Source: CAD feature listing. Evaluate the final solid. Frame: model axes, mm. Give positions to 0.01 mm unless a question says otherwise; leave off trailing zeros. Loops run counter-clockwise (first coordinate to the right, second up) from the corner with the lowest first, then second, coordinate; pieces in that order, holes last. Notation, with made-up numbers: M 45,-13.75 L 56,-13.75 A12 ccw 56,1.25 Z; hole C 50,-2 d11. An arc over 180 degrees is marked long. Put each result on its own line as item: value. Start each with the question number.
```python
from build123d import *

# Parameters (mm, degrees)
SKETCH1_R           = 3.5
BOSS_EXTRUDE1_DEPTH = 15
BOSS_EXTRUDE1_TAPER = 4


with BuildPart() as part:
    # Sketch1 → Boss-Extrude1 (new body)
    with BuildSketch(Plane(origin=(0, 0, 0), x_dir=(0, 0, -1), z_dir=(1, 0, 0))):
        Circle(SKETCH1_R)
    extrude(amount=BOSS_EXTRUDE1_DEPTH, taper=BOSS_EXTRUDE1_TAPER)

    # Sketch2 → Revolve1 (revolve)
    with BuildSketch(Plane(origin=(16, 0, 0), x_dir=(0, 0, -1), z_dir=(1, 0, 0))):
        with BuildLine():
            Line((0, 2.451097821), (0, -2.451097821))
            ThreePointArc((0, -2.451097821), (2.451097821, 0), (0, 2.451097821))
        make_face()
    revolve(axis=Axis((16, 2.451097821, 0), (0, -1, 0)))


solid = part.part
```
1. Section B-B, the plane x = 10.75. Output: boundary loops of the cut face in (y, z), plus the area to 3 significant figures.
2. Section A-A, the plane z = 0. Output: boundary loops of the cut face in (x, y).
3. Ray query, line 1 (Z direction, x = 4.75, y = 2); line 2 (Z direction, x = 2.5, y = -0.25); line 3 (Y direction, x = 15.75, z = 2). Return the intervals inside material, ascending.
4. Section C-C, the plane x = 4.25. Output: boundary loops of the cut face in (y, z), plus the area to 3 significant figures.
5. Contact query for flat-ended pins moving along their axis: pin 1 (3 mm diameter, centred on x = 4, z = 2.5, fed in from +Y); pin 2 (1.5 mm diameter, centred on y = 0.5, z = -1, fed in from +X); pin 3 (3 mm diameter, centred on x = 7.5, y = 0.5, fed in from +Z). Output: stop coordinate, or through.
Results found:
1. outline: C 0,0 d5.5
1. area: 23.7 mm²
2. outline: M 0,-3.5 L 15,-2.45 L 15,-2.24 A2.45 ccw long 15,2.24 L 15,2.45 L 0,3.5 Z
3. line 1: -2.46 to 2.46
3. line 2: -3.32 to 3.32
3. line 3: -1.39 to 1.39
4. outline: C 0,0 d6.41
4. area: 32.2 mm²
5. pin 1: y = 3.07
5. pin 2: x = 18.42
5. pin 3: z = 3.08
